Answer from the drawing. Dimensions are ordinates in mm from the lowest x, y and z of the part. Give positions to 0.01 mm unless a question says otherwise; leave off trailing zeros. Loops run counter-clockwise (first coordinate to the right, second up) from the corner with the lowest first, then second, coordinate; pieces in that order, holes last. Notation, with made-up numbers: (63, -7.75) -> (88, -7.75) arc R23 ccw to (88, 30.25) -> close; hole circle Ø11 at (21.5, 68). An arc over 180 degrees is marked (long way). Write each question's results on one line, items separated by ' | '. Start each with the question number.
Item 1: Section B-B on x = 77.5 is taken. Write down the section's boundary in (y, z) (3 decimals).
Item 2: Section A-A on z = 10 is taken. Write down the section's boundary in (x, y) (1 decimal).
Item 3: Find the intervals of material crossed by line 1 (Z direction, x = 50.8, y = 202.5) (3 decimals); line 2 (X direction, y = 18.5, z = 50.5); line 3 (X direction, y = 165, z = 71.5), in increasing order.
Item 4: Each of these flat-tipped pins is pushed along its axis until it touches: P1, Ø10, axis at y = 68.5, z = 80.5, coming from the +X side; P2, Ø3, axis at y = 203.2, z = 50.8, coming from the -X side; P3, Ø6, axis at y = 39, z = 62.5, coming from the -X side. Where does it stop, or does it pass through?
Item 5: Determine the mould class of the marked faces 1 and 2 for opening direction Z: +Z half, -Z half, draft (parallel to the pull), parting line (faces both ways), or undercut.
Item 6: Section C-C on y = 166 is taken. Write down the section's boundary in (x, z) (3 decimals).
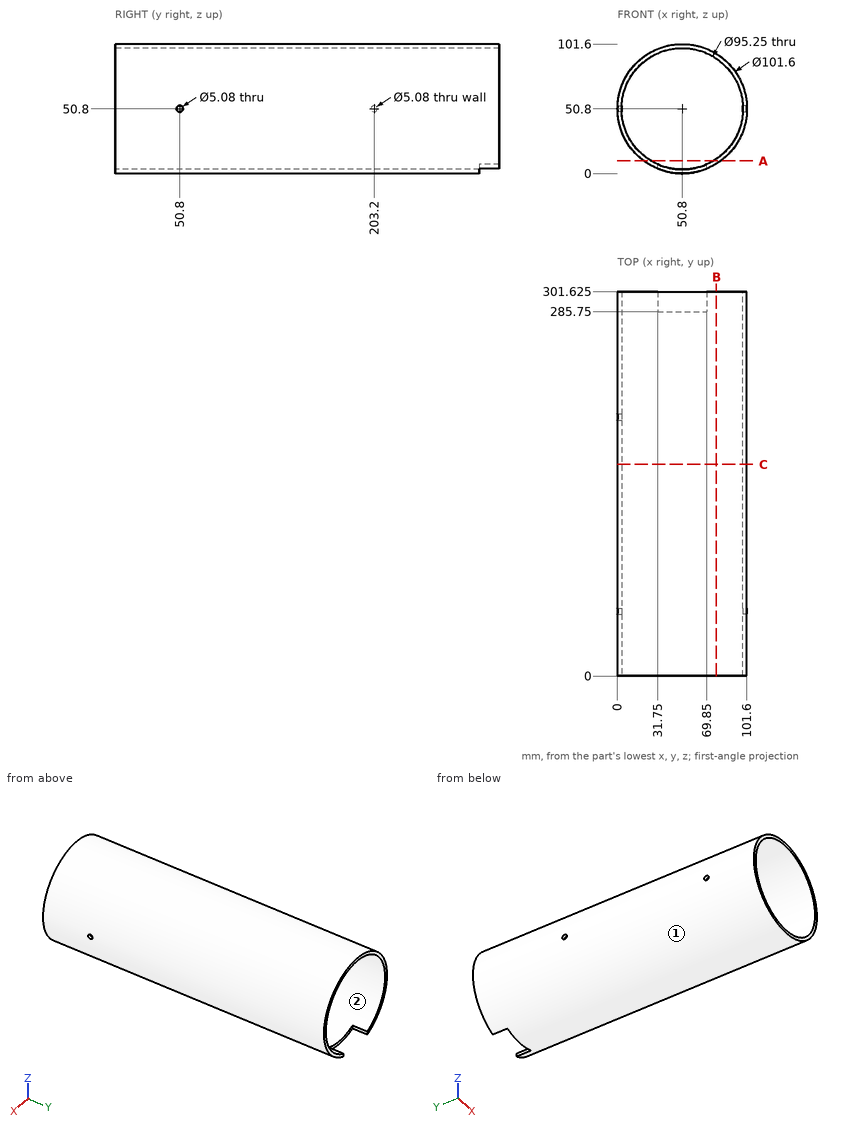
Findings:
1) outline: (0, 7.583) -> (301.625, 7.583) -> (301.625, 11.363) -> (0, 11.363) -> close; (0, 90.237) -> (301.625, 90.237) -> (301.625, 94.017) -> (0, 94.017) -> close
2) outline: (20.5, 0) -> (26.2, 0) -> (26.2, 301.6) -> (20.5, 301.6) -> close; (75.4, 0) -> (81.1, 0) -> (81.1, 301.6) -> (75.4, 301.6) -> close
3) line 1: 0 to 3.175, 98.425 to 101.6 | line 2: 0 to 3.18, 98.42 to 101.6 | line 3: 4.41 to 7.91, 93.69 to 97.19
4) P1: x = 95.19 | P2: x = 98.4 | P3: x = 0.75
5) face 1: parting line | face 2: undercut
6) outline: circle Ø101.6 at (50.8, 50.8); hole circle Ø95.25 at (50.8, 50.8)
